Here's how the part is built. I have some questions about the finished solid (model axes, mm). A direction names the side the tool comes from. Give positions to 0.01 mm unless a question says otherwise; leave off trailing zeros. Order: outer loops, then holes, each group sorted by start corner. A loop starts at its lowest first (then second) coordinate and runs counter-clockwise, first axis right, second up.
from build123d import *

# Parameters (mm, degrees)
SKETCH_1_W          = 40
SKETCH_1_H          = 38
SKETCH_1_R          = 5
EXTRUDE_1_DEPTH     = 2.5
EXTRUDE_2_DEPTH     = 14
SKETCH_3_R          = 4.25
CUT_EXTRUDE_2_DEPTH = 3
SKETCH_4_W          = 2
SKETCH_4_H          = 11.937460889
SKETCH_4_H_2        = 38
EXTRUDE_3_DEPTH     = 40
CUT_EXTRUDE_3_REACH = 42
SKETCH_5_R          = 1.75
SKETCH_5_R_2        = 4.25


with BuildPart() as part:
    # 草图1 → 凸台-拉伸1 (new body)
    with BuildSketch(Plane.XY):
        Rectangle(SKETCH_1_W, SKETCH_1_H)
        Circle(SKETCH_1_R, mode=Mode.SUBTRACT)
    extrude(amount=EXTRUDE_1_DEPTH)

    # 草图2 → 凸台-拉伸2 (add)
    with BuildSketch(Plane.XY.offset(2.5)):
        Polygon((-18, 19), (-18, -19), (-20, -19), (-20, 19), (-20, 31), (-18, 31), align=None)
    extrude(amount=EXTRUDE_2_DEPTH)

    # 草图3 → 切除-拉伸2 (cut, through all)
    with BuildSketch(Plane(origin=(-18, 0, 0), x_dir=(0, 0, -1), z_dir=(1, 0, 0))):
        with BuildLine():
            Line((-16.5, -19), (-6.5, -19))
            ThreePointArc((-6.5, -19), (-13.571067812, -16.071067812), (-16.5, -9))
            Line((-16.5, -9), (-16.5, -19))
        make_face()
        with BuildLine():
            Line((-16.5, 31), (-16.5, 24))
            ThreePointArc((-16.5, 24), (-14.449747468, 28.949747468), (-9.5, 31))
            Line((-9.5, 31), (-16.5, 31))
        make_face()
        with BuildLine():
            ThreePointArc((-9.5, 31), (-4.550252532, 28.949747468), (-2.5, 24))
            Line((-2.5, 24), (-2.5, 31))
            Line((-2.5, 31), (-9.5, 31))
        make_face()
        with Locations((-9.5, 24)):
            Circle(SKETCH_3_R)
    extrude(amount=-CUT_EXTRUDE_2_DEPTH, mode=Mode.SUBTRACT)

    # 草图4 → 凸台-拉伸3 (add)
    with BuildSketch(Plane.XY.offset(2.5)):
        with Locations((19, 24.968730445)):
            Rectangle(SKETCH_4_W, SKETCH_4_H)
        with Locations((19, 0)):
            Rectangle(SKETCH_4_W, SKETCH_4_H_2)
    extrude(amount=EXTRUDE_3_DEPTH)

    # 草图5 → 切除-拉伸3 (cut, up to next)
    with BuildSketch(Plane(origin=(20, 0, 0), x_dir=(0, 0, -1), z_dir=(1, 0, 0)), mode=Mode.PRIVATE) as cut_extrude_3_sk1:
        with BuildLine():
            ThreePointArc((-35.5, -14), (-40.449747452, -11.949747484), (-42.5, -7.000000045))
            Line((-42.5, -7.000000045), (-42.5, -19))
            Line((-42.5, -19), (-16.5, -19))
            Line((-16.5, -19), (-16.5, -18.915955378))
            ThreePointArc((-16.5, -18.915955378), (-17.129495713, -18.813310688), (-17.751167584, -18.670745373))
            Line((-17.751167584, -18.670745373), (-35.5, -14))
        make_face()
    cut_extrude_3_tool1 = extrude(cut_extrude_3_sk1.sketch, amount=-CUT_EXTRUDE_3_REACH, mode=Mode.PRIVATE) & part.part
    add(cut_extrude_3_tool1.solids().sort_by_distance((20, -16.467085, 34.190758))[0], mode=Mode.SUBTRACT)
    # 草图5 → 切除-拉伸3 (cut, up to next)
    with BuildSketch(Plane(origin=(20, 0, 0), x_dir=(0, 0, -1), z_dir=(1, 0, 0)), mode=Mode.PRIVATE) as cut_extrude_3_sk2:
        with BuildLine():
            ThreePointArc((-16.5, 24), (-14.769502014, 28.60785726), (-10.433614706, 30.937460889))
            Line((-10.433614706, 30.937460889), (-42.5, 30.937460889))
            Line((-42.5, 30.937460889), (-42.5, -7.000000045))
            ThreePointArc((-42.5, -7.000000045), (-40.449747484, -2.050252548), (-35.5, 0))
            Line((-35.5, 0), (-22.492126933, 5.690411164))
            ThreePointArc((-22.492126933, 5.690411164), (-18.131047537, 9.37849159), (-16.5, 14.852122439))
            Line((-16.5, 14.852122439), (-16.5, 24))
        make_face()
    cut_extrude_3_tool2 = extrude(cut_extrude_3_sk2.sketch, amount=-CUT_EXTRUDE_3_REACH, mode=Mode.PRIVATE) & part.part
    add(cut_extrude_3_tool2.solids().sort_by_distance((20, 16.838407, 30.295804))[0], mode=Mode.SUBTRACT)
    # 草图5 → 切除-拉伸3 (cut, up to next)
    with BuildSketch(Plane(origin=(20, 0, 0), x_dir=(0, 0, -1), z_dir=(1, 0, 0)), mode=Mode.PRIVATE) as cut_extrude_3_sk3:
        with BuildLine():
            Line((-2.5, 24), (-2.5, 25))
            Line((-2.5, 25), (-2.5, 30.937460889))
            Line((-2.5, 30.937460889), (-8.566385294, 30.937460889))
            ThreePointArc((-8.566385294, 30.937460889), (-4.230497986, 28.60785726), (-2.5, 24))
        make_face()
    cut_extrude_3_tool3 = extrude(cut_extrude_3_sk3.sketch, amount=-CUT_EXTRUDE_3_REACH, mode=Mode.PRIVATE) & part.part
    add(cut_extrude_3_tool3.solids().sort_by_distance((20, 29.375995, 3.999369))[0], mode=Mode.SUBTRACT)
    # 草图5 → 切除-拉伸3 (cut, up to next)
    with BuildSketch(Plane(origin=(20, 0, 0), x_dir=(0, 0, -1), z_dir=(1, 0, 0)), mode=Mode.PRIVATE) as cut_extrude_3_sk4:
        with Locations((-35.5, -7)):
            Circle(SKETCH_5_R)
    cut_extrude_3_tool4 = extrude(cut_extrude_3_sk4.sketch, amount=-CUT_EXTRUDE_3_REACH, mode=Mode.PRIVATE) & part.part
    add(cut_extrude_3_tool4.solids().sort_by_distance((20, -7, 35.5))[0], mode=Mode.SUBTRACT)
    # 草图5 → 切除-拉伸3 (cut, up to next)
    with BuildSketch(Plane(origin=(20, 0, 0), x_dir=(0, 0, -1), z_dir=(1, 0, 0)), mode=Mode.PRIVATE) as cut_extrude_3_sk5:
        with Locations((-9.5, 24)):
            Circle(SKETCH_5_R_2)
    cut_extrude_3_tool5 = extrude(cut_extrude_3_sk5.sketch, amount=-CUT_EXTRUDE_3_REACH, mode=Mode.PRIVATE) & part.part
    add(cut_extrude_3_tool5.solids().sort_by_distance((20, 24, 9.5))[0], mode=Mode.SUBTRACT)


solid = part.part
Q1. If we section it at A-A on x = 0: List the corners of the cut face in (y, z) for me, plus the area to 3 significant figures.
Filled sheet:
outline: (-19, 0) - (-5, 0) - (-5, 2.5) - (-19, 2.5) - close; (5, 0) - (19, 0) - (19, 2.5) - (5, 2.5) - close
area: 70.0 mm2
Q2. For faces 4 (the face through (18, 1, 18)), 5 (the face through (1, -19, 2)), 6 (the face through (19, 19, 16.5)), 7 (the face through (-18.99, -16.15, 13.49)), 8 (the face through (19, 22, 2.5)), which set-ups out of +Z, -Z, +X, -X, +Y, -Y let a thin tool reach every point of the face, with its end or its side?
Filled sheet:
face 4: +Z, +Y, -Y
face 5: +Z, -Z, +X, -X, -Y
face 6: +Z, +X, -X, +Y
face 7: +Z, -X, -Y
face 8: -Z, +X, -X, +Y
Q3. If we section it at C-C on y = 2: List the corners of the cut face in (x, z) for me.
Filled sheet:
outline: (-20, 0) - (-4.58, 0) - (-4.58, 2.5) - (-18, 2.5) - (-18, 16.5) - (-20, 16.5) - close; (4.58, 0) - (20, 0) - (20, 30.93) - (18, 30.93) - (18, 2.5) - (4.58, 2.5) - close
Q4. I need wall thicknesses on L1, parallel to X at y = 15, z = 11; L2, parallel to Y at x = 0, z = 1; L3, parallel to Z at x = -13.5, y = -10. Which ranges of each line are inside material? Lowest first, please.
Filled sheet:
L1: x = -20 to -18, 18 to 20
L2: y = -19 to -5, 5 to 19
L3: z = 0 to 2.5
Q5. If we section it at B-B on y = 21.5: List the corners of the cut face in (x, z) for me, plus the area to 3 significant figures.
Filled sheet:
outline: (-20, 2.5) - (-18, 2.5) - (-18, 6.06) - (-20, 6.06) - close; (-20, 12.94) - (-18, 12.94) - (-18, 16.5) - (-20, 16.5) - close; (18, 2.5) - (20, 2.5) - (20, 6.06) - (18, 6.06) - close; (18, 12.94) - (20, 12.94) - (20, 16.5) - (18, 16.5) - close
area: 28.5 mm2
Q6. Thinking about a two-plate mould opening in Y: for faces 1 (the face through (19.014, 28.661, 4.277)), 2 (the face through (19.014, 27.584, 7.215)), 3 (the face through (-4, 4, 2.5)), which applies, released by +Y, released by -Y, zero draft, split by the parting line, or undercut?
Filled sheet:
face 1: released by +Y
face 2: undercut
face 3: zero draft
Q7. I'm going to push flat-ended pins straight in: P1, Ø1.2, axis at x = -3, z = 1.5, coming from the +Y side; P2, Ø2, axis at x = 18.5, y = 20.5, coming from the -Z side; P3, Ø7.5, axis at y = 24, z = 9.5, coming from the +X side; P4, Ø1.5, axis at y = 4, z = 23, coming from the -X side. Where does each tip first touch, or does it pass through?
Filled sheet:
P1: stops at y = 19
P2: stops at z = 2.5
P3: passes through
P4: stops at x = 18
Q8. If we section it at D-D on z = 38: List the corners of the cut face in (x, y) for me.
Filled sheet:
outline: (18, -13.54) - (20, -13.54) - (20, -0.46) - (18, -0.46) - close
